The listing builds one solid part. Answer for the finished solid, in the listing's coordinates (mm). A direction names the side the tool comes from. Coordinates: 2 decimals unless noted, no trailing zeros. Order: outer loops, then holes, each group sorted by start corner. A loop starts at its lowest first (then second) coordinate and runs counter-clockwise, first axis right, second up. Notation, with made-up numbers: (4.25, 28.5) -> (39.25, 28.5) arc R21 cw to (39.25, 42.5) -> close; hole circle Ø1 at (-13.5, 81). An arc over 180 degrees is marked (long way). Write each question's results on one line, items separated by ' | '. Start each with the question number.
(1) The part is cut by section B-B, the plane y = -14.5. Give the vertices of the cut face in (x, z), then the cut area to 3 significant figures.
(2) Determine the mould class of faces 5 (the face through (15, -33.781, -32)), 6 (the face through (2, -22, -63.462)), 7 (the face through (10, -6.331, -38)) for opening direction Y: +Y half, -Y half, draft (parallel to the pull), parting line (faces both ways), or undercut.
(3) The part is cut by section A-A, the plane z = -3.5. Give the vertices of the cut face in (x, y), then the cut area to 3 significant figures.
(4) Straight lines are drawn through the part: L1, parallel to Y at x = 25, z = -14; L2, parallel to Z at x = 27, y = -11; L3, parallel to Z at x = 14.5, y = -22. For each, find the intervals that lie inside material, in ascending order.
(5) The part is cut by section D-D, the plane y = -0.5. Give the vertices of the cut face in (x, z).
(6) A tool of negligible diameter and unlimited length cuts with its end or side. For faces 1 (the face through (11, -30.781, -45)), 2 (the face through (15, 1.969, -9)), 3 (the face through (12, -38.781, -46)), 4 (the face through (15, -5, -35.462)), from which of +Z, -Z, +X, -X, +Y, -Y can it reach the whole face along a straight path? Write none if from no direction.
(7) Given pin 1 (12 mm diameter, centred on x = 24.5, y = -2.5, fed in from -Z); pin 2 (3 mm diameter, centred on x = 1.5, z = -42, fed in from +Y); pin 3 (2 mm diameter, centred on x = 19, y = -41, fed in from +Z); pin 4 (10 mm diameter, centred on x = 20, y = -37, fed in from +Z), each flat-ended and moving along its own axis, determine where each tip first touches the part or whether it passes through.
(8) The part is cut by section C-C, the plane x = 16.5. Give the vertices of the cut face in (y, z), then the cut area to 3 significant figures.
```python
from build123d import *

# Parameters (mm, degrees)
BOSS_EXTRUDE1_DEPTH = 30
SKETCH3_R           = 4.4
CUT_EXTRUDE1_DEPTH  = 30
SKETCH4_W           = 3.511443211
SKETCH4_H           = 32.45
BOSS_EXTRUDE2_DEPTH = 25
SKETCH5_R           = 3
CUT_EXTRUDE2_DEPTH  = 20
SKETCH6_W           = 26.488556789
SKETCH6_H           = 8
BOSS_EXTRUDE3_DEPTH = 25
CUT_EXTRUDE5_DEPTH  = 8
SKETCH9_W           = 6
SKETCH9_H           = 15
CUT_EXTRUDE6_DEPTH  = 3.511443


with BuildPart() as part:
    # Sketch1 → Boss-Extrude1 (new body)
    with BuildSketch(Plane(origin=(0, 0, 0), x_dir=(0, 0, -1), z_dir=(1, 0, 0))):
        with BuildLine():
            ThreePointArc((24.712382734, 6.969258669), (32.225912197, 3.9087055), (35.462382734, -3.530741331))
            Line((35.462382734, -3.530741331), (35.462382734, -6.330741331))
            Line((35.462382734, -6.330741331), (38.462382734, -6.330741331))
            Line((38.462382734, -6.330741331), (38.462382734, -38.780741331))
            Line((38.462382734, -38.780741331), (35.035529086, -38.780741331))
            ThreePointArc((35.035529086, -38.780741331), (31.3038679, -44.275567943), (25.056259743, -46.530741331))
            Line((25.056259743, -46.530741331), (-7.537617266, -46.530741331))
            ThreePointArc((-7.537617266, -46.530741331), (-14.962238469, -43.455362534), (-18.037617266, -36.030741331))
            Line((-18.037617266, -36.030741331), (-18.037617266, -3.530741331))
            ThreePointArc((-18.037617266, -3.530741331), (-14.962238469, 3.893879871), (-7.537617266, 6.969258669))
            Line((-7.537617266, 6.969258669), (24.712382734, 6.969258669))
        make_face()
        with BuildLine():
            Line((-13.037617266, -3.530741331), (-13.037617266, -36.030741331))
            ThreePointArc((-13.037617266, -36.030741331), (-11.426704563, -39.919828628), (-7.537617266, -41.530741331))
            Line((-7.537617266, -41.530741331), (24.962382734, -41.530741331))
            ThreePointArc((24.962382734, -41.530741331), (28.865997514, -39.759198947), (30.462382734, -35.780741331))
            Line((30.462382734, -35.780741331), (30.462382734, -33.780741331))
            Line((30.462382734, -33.780741331), (33.462382734, -33.780741331))
            Line((33.462382734, -33.780741331), (33.462382734, -11.330741331))
            Line((33.462382734, -11.330741331), (30.462382734, -11.330741331))
            Line((30.462382734, -11.330741331), (30.462382734, -3.530741331))
            ThreePointArc((30.462382734, -3.530741331), (28.69084035, 0.372873449), (24.712382734, 1.969258669))
            Line((24.712382734, 1.969258669), (-7.537617266, 1.969258669))
            ThreePointArc((-7.537617266, 1.969258669), (-11.426704563, 0.358345965), (-13.037617266, -3.530741331))
        make_face(mode=Mode.SUBTRACT)
    extrude(amount=BOSS_EXTRUDE1_DEPTH)

    # Sketch3 → Cut-Extrude1 (cut)
    with BuildSketch(Plane(origin=(0, 0, -38.462382734), x_dir=(-1, 0, 0), z_dir=(0, 0, -1))):
        with Locations((-8.5, -19.730741331)):
            Circle(SKETCH3_R)
    extrude(amount=-CUT_EXTRUDE1_DEPTH, mode=Mode.SUBTRACT)

    # Sketch4 → Boss-Extrude2 (add)
    with BuildSketch(Plane(origin=(0, 0, -38.462382734), x_dir=(-1, 0, 0), z_dir=(0, 0, -1))):
        with Locations((-1.755721606, -22.555741331)):
            Rectangle(SKETCH4_W, SKETCH4_H)
    extrude(amount=BOSS_EXTRUDE2_DEPTH)

    # Sketch5 → Cut-Extrude2 (cut)
    with BuildSketch(Plane(origin=(3.511443211, 0, 0), x_dir=(0, 0, -1), z_dir=(1, 0, 0))):
        with Locations((53.462382734, -22.639729025)):
            Circle(SKETCH5_R)
    extrude(amount=-CUT_EXTRUDE2_DEPTH, mode=Mode.SUBTRACT)

    # Sketch6 → Boss-Extrude3 (add)
    with BuildSketch(Plane(origin=(0, 0, -38.462382734), x_dir=(-1, 0, 0), z_dir=(0, 0, -1))):
        with Locations((-16.755721606, -34.780741331)):
            Rectangle(SKETCH6_W, SKETCH6_H)
    extrude(amount=BOSS_EXTRUDE3_DEPTH)

    # Sketch8 → Cut-Extrude5 (cut)
    with BuildSketch(Plane(origin=(0, -30.780741331, 0), x_dir=(1, 0, 0), z_dir=(0, 1, 0))):
        Polygon((3.511443211, 63.462382734), (30, 38.462382734), (30, 63.462382734), align=None)
    extrude(amount=-CUT_EXTRUDE5_DEPTH, mode=Mode.SUBTRACT)

    # Sketch9 → Cut-Extrude6 (cut)
    with BuildSketch(Plane(origin=(3.511443211, 0, 0), x_dir=(0, 0, -1), z_dir=(1, 0, 0))):
        with Locations((41.462382734, -20.113548678)):
            Rectangle(SKETCH9_W, SKETCH9_H)
    extrude(amount=-CUT_EXTRUDE6_DEPTH, mode=Mode.SUBTRACT)


solid = part.part
```
Established:
1) outline: (0, -63.46) -> (3.51, -63.46) -> (3.51, -44.46) -> (0, -44.46) -> close; (0, -38.46) -> (30, -38.46) -> (30, -33.46) -> (0, -33.46) -> close; (0, 13.04) -> (30, 13.04) -> (30, 18.04) -> (0, 18.04) -> close | area: 367 mm^2
2) face 5: undercut | face 6: draft | face 7: +Y half
3) outline: (0, -46.53) -> (30, -46.53) -> (30, -41.53) -> (0, -41.53) -> close; (0, 1.97) -> (30, 1.97) -> (30, 6.97) -> (0, 6.97) -> close | area: 300 mm^2
4) L1: y = -46.53 to -41.53, 1.97 to 6.97 | L2: z = -38.46 to -30.46, 13.04 to 18.04 | L3: z = -38.46 to -33.46, 13.04 to 18.04
5) outline: (0, -34.95) -> (30, -34.95) -> (30, -29.44) -> (0, -29.44) -> close; (0, 12.13) -> (30, 12.13) -> (30, 17.59) -> (0, 17.59) -> close
6) face 1: -Z, +X, +Y | face 2: +X, -X | face 3: -Z, +X, -X, -Y | face 4: -Z, +X, -X, +Y
7) pin 1: stops at z = -38.46 | pin 2: stops at y = -6.33 | pin 3: stops at z = 17.26 | pin 4: stops at z = 18.04
8) outline: (-46.53, -25.06) arc R10.76 ccw to (-38.78, -35.04) -> (-38.78, -51.2) -> (-30.78, -51.2) -> (-30.78, -38.46) -> (-6.33, -38.46) -> (-6.33, -35.46) -> (-3.53, -35.46) arc R10.75 ccw to (6.97, -24.71) -> (6.97, 7.54) arc R10.5 ccw to (-3.53, 18.04) -> (-36.03, 18.04) arc R10.5 ccw to (-46.53, 7.54) -> close; hole (-41.53, -24.96) arc R5.76 ccw to (-35.78, -30.46) -> (-33.78, -30.46) -> (-33.78, -33.46) -> (-11.33, -33.46) -> (-11.33, -30.46) -> (-3.53, -30.46) arc R5.76 ccw to (1.97, -24.71) -> (1.97, 7.54) arc R5.5 ccw to (-3.53, 13.04) -> (-36.03, 13.04) arc R5.5 ccw to (-41.53, 7.54) -> close | area: 1,030 mm^2
